```python
from build123d import *

# Parameters (mm, degrees)
SKETCH1_W           = 40
SKETCH1_H           = 42
BOSS_EXTRUDE1_DEPTH = 2
SKETCH2_W           = 40
SKETCH2_H           = 2
BOSS_EXTRUDE2_DEPTH = 50
CUT_EXTRUDE1_DEPTH  = 50
SKETCH4_R           = 1.5
CUT_EXTRUDE2_DEPTH  = 50
CUT_EXTRUDE3_DEPTH  = 1033
SKETCH6_R           = 1.5
CUT_EXTRUDE4_DEPTH  = 1033


with BuildPart() as part:
    # Sketch1 → Boss-Extrude1 (new body)
    with BuildSketch(Plane(origin=(0, 0, 0), x_dir=(1, 0, 0), z_dir=(0, 1, 0))):
        Rectangle(SKETCH1_W, SKETCH1_H)
    extrude(amount=BOSS_EXTRUDE1_DEPTH)

    # Sketch2 → Boss-Extrude2 (add)
    with BuildSketch(Plane(origin=(0, 2, 0), x_dir=(1, 0, 0), z_dir=(0, 1, 0))):
        with Locations((0, -20)):
            Rectangle(SKETCH2_W, SKETCH2_H)
    extrude(amount=BOSS_EXTRUDE2_DEPTH)

    # Sketch3 → Cut-Extrude1 (cut)
    with BuildSketch(Plane.XY.offset(21)):
        with BuildLine():
            Line((-20, 52), (-20, 32))
            ThreePointArc((-20, 32), (-14.142135619, 46.142135629), (1.4e-08, 52))
            Line((1.4e-08, 52), (-20, 52))
        make_face()
        with BuildLine():
            Line((20, 52), (1.4e-08, 52))
            ThreePointArc((1.4e-08, 52), (14.142135629, 46.142135619), (20, 32))
            Line((20, 32), (20, 52))
        make_face()
    extrude(amount=-CUT_EXTRUDE1_DEPTH, mode=Mode.SUBTRACT)

    # Sketch4 → Cut-Extrude2 (cut)
    with BuildSketch(Plane.XY.offset(21)):
        with Locations((-15.5, 32)):
            Circle(SKETCH4_R)
        with Locations((15.5, 32)):
            Circle(SKETCH4_R)
        with Locations((7.75, 18.576606241)):
            Circle(SKETCH4_R)
        with Locations((-7.75, 18.576606241)):
            Circle(SKETCH4_R)
        with Locations((-7.75, 45.423393759)):
            Circle(SKETCH4_R)
        with Locations((7.75, 45.423393759)):
            Circle(SKETCH4_R)
    extrude(amount=-CUT_EXTRUDE2_DEPTH, mode=Mode.SUBTRACT)

    # Sketch5 → Cut-Extrude3 (cut)
    with BuildSketch(Plane.XY.offset(21)):
        with BuildLine():
            ThreePointArc((6, 51.078784028), (0, 52), (-6, 51.078784028))
            Line((-6, 51.078784028), (-6, 19))
            ThreePointArc((-6, 19), (0, 13), (6, 19))
            Line((6, 19), (6, 51.078784028))
        make_face()
    extrude(amount=-CUT_EXTRUDE3_DEPTH, mode=Mode.SUBTRACT)

    # Sketch6 → Cut-Extrude4 (cut)
    with BuildSketch(Plane.XZ):
        with Locations(Location((-10, 9.5, 0), (0, 0, 270))):
            Circle(SKETCH6_R)
        with Locations(Location((10, 9.5, 0), (0, 0, 270))):
            Circle(SKETCH6_R)
        with Locations(Location((10, -10.5, 0), (0, 0, 270))):
            Circle(SKETCH6_R)
        with Locations(Location((-10, -10.5, 0), (0, 0, 270))):
            Circle(SKETCH6_R)
    extrude(amount=-CUT_EXTRUDE4_DEPTH, mode=Mode.SUBTRACT)


solid = part.part
```
Input: part model. Units: mm. Frame: model coordinates. A direction names the side the tool comes from. Give positions to 0.01 mm unless a question says otherwise; leave off trailing zeros. Write each loop counter-clockwise with the first axis right and the second up, starting at its lowest first coordinate (ties: lowest second). Pieces come first, ordered by that corner, then holes. Notation, with made-up numbers: (-2.75, 86.25) - (13.25, 86.25) arc R25 cw to (13.25, 111.25) - close; hole circle Ø2 at (64, 23). An arc over 180 degrees is marked (long way). Write item = value, one per line. Start each with the question number.
1. Section query A-A, the plane y = 48. Output: boundary loops of the cut face in (x, z), then the cut area to 3 significant figures.
2. Access query for faces 1 (the flat face through (0, 2, -1)), 2 (the cylindrical face through (-9.25, 18.64, 20.01)), 3 (the flat face through (6, 35, 20)). Directions: +Z, -Z, +X, -X, +Y, -Y. A direction counts if a zero-diameter tool reaches every point of the face in a straight line with its end or side. Return the directions, or none.
3. First-contact query: pin 1 Ø2.5 at (x, z) = (10, -10.5) entering from +Y; pin 2 Ø6 at (x, z) = (-15.5, 6.5) entering from +Y; pin 3 Ø2 at (y, z) = (42, 20) entering from -X. Flat tips, straight axial feed; report the tip coordinate or a pass-through.
4. Ray query, L1, parallel to X at y = 1.5, z = 9.5; L2, parallel to Y at x = 4, z = 5; L3, parallel to Y at x = 7.75, z = 19.8. Return the intervals inside material, ascending.
5. Section query D-D, the plane x = -15.5. Output: boundary loops of the cut face in (y, z), then the cut area to 3 significant figures.
6. Section query C-C, the plane x = -7.75. Output: boundary loops of the cut face in (y, z).
7. Mould query, pull axis X, two halves, no side actions, for faces 4 (the cylindrical face through (-8.856, 46.437, 20.014)), 5 (the cylindrical face through (16, 44, 20)), 6 (the cylindrical face through (-16, 44, 20)). Classes: released by +X, released by -X, zero draft, split by the parting line, or undercut.
8. Section query B-B, the plane z = -10.5. Output: boundary loops of the cut face in (x, y), then the cut area to 3 significant figures.
Check sheet entries:
q1.outline = (-12, 19) - (-6, 19) - (-6, 21) - (-12, 21) - close; (6, 19) - (12, 19) - (12, 21) - (6, 21) - close
q1.area = 24.0 mm2
q2.face_1 = -Z, +X, -X, +Y
q2.face_2 = +Z, -Z
q2.face_3 = +Z, -Z, +Y
q3.pin_1 = through
q3.pin_2 = 2
q3.pin_3 = -17.86
q4.L1 = -20 to -11.5, -8.5 to 8.5, 11.5 to 20
q4.L2 = 0 to 2
q4.L3 = 0 to 17.08, 20.08 to 43.92, 46.92 to 50.44
q5.outline = (0, -21) - (2, -21) - (2, 19) - (30.5, 19) - (30.5, 21) - (0, 21) - close; (33.5, 19) - (44.64, 19) - (44.64, 21) - (33.5, 21) - close
q5.area = 163 mm2
q6.outline = (0, -21) - (2, -21) - (2, 19) - (17.08, 19) - (17.08, 21) - (0, 21) - close; (20.08, 19) - (43.92, 19) - (43.92, 21) - (20.08, 21) - close; (46.92, 19) - (50.44, 19) - (50.44, 21) - (46.92, 21) - close
q7.face_4 = undercut
q7.face_5 = released by +X
q7.face_6 = released by -X
q8.outline = (-20, 0) - (-11.5, 0) - (-11.5, 2) - (-20, 2) - close; (-8.5, 0) - (8.5, 0) - (8.5, 2) - (-8.5, 2) - close; (11.5, 0) - (20, 0) - (20, 2) - (11.5, 2) - close
q8.area = 68.0 mm2
